Check sheet for the modelled part. Datum: model origin and axes. Units: mm. A direction names the side the tool comes from. Round coordinates to 2 decimals unless told otherwise and drop trailing zeros. Write each loop counter-clockwise with the first axis right and the second up, starting at its lowest first coordinate (ties: lowest second). Pieces come first, ordered by that corner, then holes. Notation, with made-up numbers: M 50,-37.75 L 90,-37.75 A29 cw 90,-1.75 Z; hole C 0,-19 d10. An arc over 180 degrees is marked long. Answer in a Markdown table with one row per item.
```python
from build123d import *

# Parameters (mm, degrees)
SKETCH1_R                       = 73.63206
SKETCH1_R_2                     = 9.525
SKETCH1_R_3                     = 7.14375
BOSS_EXTRUDE1_DEPTH             = 6.35
CIRPATTERN1_COUNT               = 2
CIRPATTERN1_ANGLE               = 90
CIRPATTERN1_THE_OTHER_WAY_COUNT = 2
CIRPATTERN1_THE_OTHER_WAY_ANGLE = 90
SKETCH1_4_R                     = 9.525
SKETCH1_4_R_2                   = 7.14375
CUT_EXTRUDE2_DEPTH              = 3.175
CIRPATTERN2_COUNT               = 12


with BuildPart() as part:
    # Sketch1 → Boss-Extrude1 (new body)
    with BuildSketch(Plane(origin=(0, 0, 0), x_dir=(1, 0, 0), z_dir=(0, 1, 0))):
        Circle(SKETCH1_R)
        Circle(SKETCH1_R_2, mode=Mode.SUBTRACT)
        Circle(SKETCH1_R_2)
        Circle(SKETCH1_R_3, mode=Mode.SUBTRACT)
    extrude(amount=BOSS_EXTRUDE1_DEPTH)

    # Sketch2 → Nozzle (revolve, cut)
    with BuildSketch(Plane(origin=(63.53048, 0, 0), x_dir=(0, 0, -1), z_dir=(1, 0, 0))):
        Polygon((-17.960512242, -11.610512242), (17.960512242, 24.310512242), (17.170249703, 25.100774781), (-3.330262539, 4.600262539), (-22.882688583, -6.688335901), align=None)
    nozzle = revolve(axis=Axis((63.53048, 24.310512242, -17.960512242), (0, -0.707106781, 0.707106781)), mode=Mode.SUBTRACT)

    # CirPattern1: Nozzle ×2 about axis
    cirpattern1_axis = Axis((0, 6.35, 0), (0, -1, 0))
    for i in range(1, CIRPATTERN1_COUNT):
        add(nozzle.rotate(cirpattern1_axis, i * CIRPATTERN1_ANGLE / (CIRPATTERN1_COUNT - 1)), mode=Mode.SUBTRACT)

    # CirPattern1 the other way: Nozzle ×2 about axis
    cirpattern1_the_other_way_axis = Axis((0, 6.35, 0), (0, 1, 0))
    for i in range(1, CIRPATTERN1_THE_OTHER_WAY_COUNT):
        add(nozzle.rotate(cirpattern1_the_other_way_axis, i * CIRPATTERN1_THE_OTHER_WAY_ANGLE / (CIRPATTERN1_THE_OTHER_WAY_COUNT - 1)), mode=Mode.SUBTRACT)

    # Sketch1_4 → Cut-Extrude2 (cut)
    with BuildSketch(Plane(origin=(0, 0, 0), x_dir=(1, 0, 0), z_dir=(0, 1, 0))):
        Circle(SKETCH1_4_R)
        Circle(SKETCH1_4_R_2, mode=Mode.SUBTRACT)
    extrude(amount=CUT_EXTRUDE2_DEPTH, mode=Mode.SUBTRACT)

    # Sketch5 → CBORE for _10 Binding Head Machine Screw (revolve, cut)
    with BuildSketch(Plane(origin=(53.975, 0, 0), x_dir=(0, 0, -1), z_dir=(1, 0, 0))):
        Polygon((0, 0), (0, 15.503816902), (2.5527, 13.97), (2.5527, 3.1242), (5.55625, 3.1242), (5.55625, 0), align=None)
    cbore_for_10_binding_head_machine_screw = revolve(axis=Axis((53.975, -6.35, 0), (0, 1, 0)), mode=Mode.SUBTRACT)

    # CirPattern2: CBORE for _10 Binding Head Machine Screw ×12 about axis, 5 skipped
    cirpattern2_axis = Axis((0, 0, 0), (0, -1, 0))
    add([cbore_for_10_binding_head_machine_screw.rotate(cirpattern2_axis, i * 360 / CIRPATTERN2_COUNT) for i in range(1, CIRPATTERN2_COUNT) if i not in (4, 5, 6, 7, 8)], mode=Mode.SUBTRACT)


solid = part.part
```
1. Scan lines: L1, parallel to Z at x = 0, y = 1.35 (3 decimals); L2, parallel to X at y = 3.8, z = 0; L3, parallel to Z at x = 2, y = 2.25. Record each from-to range of solid material in increasing order.
Found:
| item | result |
|---|---|
| L1 | z = -73.632 to -59.531, -48.419 to -9.525, 9.525 to 48.419, 59.531 to 73.632 |
| L2 | x = -73.63 to -7.14, 7.14 to 51.42, 56.53 to 73.63 |
| L3 | z = -73.6 to -59.16, -48.79 to -9.31, 9.31 to 48.79, 59.16 to 73.6 |
2. Draft check along Z on faces 3 (the face through (-1, 0, 15)), 4 (the face through (-58.432, 3.131, 44.804)), 5 (the face through (47, 3.124, 30)). Enter one of: +Z half, -Z half, draft (parallel to the pull), parting line (faces both ways), or undercut.
Found:
| item | result |
|---|---|
| face 3 | draft |
| face 4 | parting line |
| face 5 | undercut |
3. Access from +Z, -Z, +X, -X, +Y, -Y to the whole of each face (thin tool, end or side, straight path). Record for faces 1 (the face through (-7.137, 4.74, -0.314)), 2 (the face through (41.444, 1.54, 28.656)).
Found:
| item | result |
|---|---|
| face 1 | +Y, -Y |
| face 2 | -Y |
4. Section check C-C, the plane z = 34.5. Record the cut outline in (x, y).
Found:
| item | result |
|---|---|
| outline | M -65.05,0 L 65.05,0 L 65.05,6.35 L -65.05,6.35 Z |
5. Section check A-A, the plane y = 1.5. Count the separate pieces of the cut face and the enclosed holes in it, and give its area (3 significant figures).
Found:
| item | result |
|---|---|
| separate pieces | 1 |
| enclosed holes | 11 |
| area | 16,000 mm2 |
6. Section check B-B, the plane x = 15. Record the cut outline in (y, z), and give its area (3 significant figures).
Found:
| item | result |
|---|---|
| outline | M 0,-72.09 L 6.35,-72.09 L 6.35,72.09 L 0,72.09 Z |
| area | 916 mm2 |
7. Go/stop test with flat-tipped pins: pin 1 (3.5 mm diameter, centred on x = 45, z = 28.5, fed in from -Y); pin 2 (1 mm diameter, centred on y = 5, z = 28, fed in from -X); pin 3 (4 mm diameter, centred on x = 53.975, z = 0, fed in from -Y); pin 4 (1 mm diameter, centred on x = -6, y = 3.5, fed in from -Z). Record where each tip stops, or that it passes through.
Found:
| item | result |
|---|---|
| pin 1 | stops at y = 3.12 |
| pin 2 | stops at x = -68.3 |
| pin 3 | passes through |
| pin 4 | stops at z = -73.43 |
